from build123d import *

# Parameters (mm, degrees)
SKETCH1_R           = 1.4
BOSS_EXTRUDE1_DEPTH = 4


with BuildPart() as part:
    # Sketch1 → Boss-Extrude1 (new body)
    with BuildSketch(Plane.XY):
        with BuildLine():
            ThreePointArc((-0.000688459, 65.016091721), (-6.500688459, 71.516091721), (-13.000688459, 65.016091721))
            Line((-13.000688459, 65.016091721), (-15.463628279, 7.853451097))
            Line((-15.463628279, 7.853451097), (-15.500688459, 6.993317296))
            ThreePointArc((-15.500688459, 6.993317296), (-5.500688459, -3.006682704), (4.499311541, 6.993317296))
            Line((4.499311541, 6.993317296), (4.379732895, 8.535158357))
            Line((4.379732895, 8.535158357), (-0.000688459, 65.016091721))
        make_face()
        with Locations((-12.500688459, 6.993317296)):
            Circle(SKETCH1_R, mode=Mode.SUBTRACT)
        with Locations((-5.500688459, 6.993317296)):
            Circle(SKETCH1_R, mode=Mode.SUBTRACT)
        with Locations((1.499311541, 6.993317296)):
            Circle(SKETCH1_R, mode=Mode.SUBTRACT)
        with Locations((-5.500688459, 26.993317296)):
            Circle(SKETCH1_R, mode=Mode.SUBTRACT)
        with Locations((-6.012756351, 45.016091721)):
            Circle(SKETCH1_R, mode=Mode.SUBTRACT)
        with Locations((-6.500688459, 65.016091721)):
            Circle(SKETCH1_R, mode=Mode.SUBTRACT)
    extrude(amount=BOSS_EXTRUDE1_DEPTH)


solid = part.part
Check sheet for the modelled part. Datum: model origin and axes. Units: mm. Give positions to 0.01 mm unless a question says otherwise; leave off trailing zeros. Loops run counter-clockwise (first coordinate to the right, second up) from the corner with the lowest first, then second, coordinate; pieces in that order, holes last. Notation, with made-up numbers: M 61,5 L 111,5 A19 ccw 111,15 Z; hole C -28,-5.75 d11. An arc over 180 degrees is marked long. Answer as a JSON object with one key per item and string values. Group by question number.
Q1. Cross-section at D-D on x = -2.5. Record the cut outline in (y, z).
Q2. Cross-section at A-A on z = 3.1. Record the cut outline in (x, y).
Q3. Release check for a two-part mould opening along Y. For faces 1 (the cylindrical face through (-6.358, 71.515, 1.972)), 2 (the cylindrical face through (-6.32, 43.65, 1.97)), 3 (the cylindrical face through (-5.721, -3.004, 1.972)) record: released by +Y, released by -Y, zero draft, split by the parting line, or undercut.
Q4. Cross-section at B-B on x = 0.75. Record the cut outline in (y, z).
Q5. Material ranges on line 1 along Y through (x, z) = (-4.25, 1.95); line 2 along X through (y, z) = (46, 0.35); line 3 along X through (y, z) = (31, 2.55), recorded low to high. Write a range as [from, to].
Q6. Go/stop test with flat-tipped pins: P1, Ø2.5, axis at x = -6.5, y = 65.02, coming from the +Z side; P2, Ø1, axis at y = 13.5, z = 1, coming from the +X side. Record where each tip stops, or that it passes through.
Q7. Cross-section at C-C on y = 51.5. Record the cut outline in (x, z).
Evaluation:
{
 "1": {"outline": "M -2.55,0 L 70.14,0 L 70.14,4 L -2.55,4 Z"},
 "2": {"outline": "M -15.5,6.99 A10 ccw 4.5,6.99 L 0,65.02 A6.5 ccw -13,65.02 Z; hole C -12.5,6.99 d2.8; hole C -6.5,65.02 d2.8; hole C -6.01,45.02 d2.8; hole C -5.5,6.99 d2.8; hole C -5.5,26.99 d2.8; hole C 1.5,6.99 d2.8"},
 "3": {"face 1": "released by +Y", "face 2": "undercut", "face 3": "released by -Y"},
 "4": {"outline": "M -0.81,0 L 5.81,0 L 5.81,4 L -0.81,4 Z; M 8.18,0 L 55.34,0 L 55.34,4 L 8.18,4 Z"},
 "5": {"line 1": "y = [-2.93, 6.36], [7.62, 26.36], [27.62, 71.11]", "line 2": "x = [-13.82, -7.01], [-5.02, 1.47]", "line 3": "x = [-14.47, 2.64]"},
 "6": {"P1": "passes through", "P2": "stops at x = 4.03"},
 "7": {"outline": "M -13.58,0 L 1.05,0 L 1.05,4 L -13.58,4 Z"}
}
